Design review of the part built by this model. Coordinates are the model's own, in mm. A direction names the side the tool comes from. Coordinates: 2 decimals unless noted, no trailing zeros. Loops run counter-clockwise (first coordinate to the right, second up) from the corner with the lowest first, then second, coordinate; pieces in that order, holes last. Notation, with made-up numbers: (29.25, -3) -> (60.25, -3) arc R34 ccw to (60.25, 30) -> close; hole circle Ø2 at (-1, 67). An arc over 180 degrees is marked (long way). One line per item, written item: value. Start each with the question number.
1. Add section C-C on y = 22. Write out the cut boundary in (x, z), plus the area to 3 significant figures.
2. Draft analysis for pull direction X (two halves, no side actions). For faces 3 (the flat face through (2, 19, 7.62)), 4 (the flat face through (-93.294, 17, 15)), 5 (the cylindrical face through (98.219, -52.015, 15.382)), 6 (the flat face through (94.666, 85, 15)), state which applies: pulls with the +X half, pulls with the -X half, needs draft (parallel to the pull), parting line crosses it, or undercut.
3. Add section B-B on x = 80.5. Write out the cut boundary in (y, z), plus the area to 3 significant figures.
4. Machinability: for faces 1 (the cylindrical face through (4.506, -52.015, 1.528)), 2 (the flat face through (4, 81.156, 6)), which of the approach directions +Z, -Z, +X, -X, +Y, -Y give a long, thin tool a straight path to every point of the face, cutting with its end or side? Answer none if there is none.
5. Add section A-A on z = 17.75. Write out the cut boundary in (x, y), plus the area to 3 significant figures.
6. Insertion check: pin 1 (1.5 mm diameter, centred on x = 50, z = 13, fed in from +Y); pin 2 (12 mm diameter, centred on x = 79, y = -39, fed in from +Z). Each pin has a flat end and moves straight along its axis. Give the tip position at first contact, or say it passes through.
7. For probe 1 along X at (y, z) = (41, 15); probe 2 along Z at (x, y) = (22, 2); probe 3 along Y at (x, z) = (36, 7.75), list the stretches that pass through material, from the lowest coordinate up.
```python
from build123d import *

# Parameters (mm, degrees)
F0_W      = 193.04
F0_H      = 142.24
F1_DEPTH  = 25.4
F2_T      = -7.62
F3_R      = 5.08
F1_FACE_W = 182.88
F1_FACE_H = 20.32
F4_DEPTH  = 7.62


with BuildPart() as f1:
    # F0 (on Top) → F1 (new body)
    with BuildSketch(Plane.XY):
        with Locations((3.226209, 17.656468)):
            Rectangle(F0_W, F0_H)
    extrude(amount=F1_DEPTH)

    # F2
    f2_openings = [f1.faces().sort_by_distance(p)[0] for p in [
        (3.226209, 17.656468, 25.4),
    ]]
    offset(amount=F2_T, openings=f2_openings)

    # F3
    f3_edges = [f1.edges().sort_by_distance(p)[0] for p in [
        (-93.293791, -53.463532, 12.7),
        (-93.293791, 88.776468, 12.7),
        (99.746209, 88.776468, 12.7),
        (99.746209, -53.463532, 12.7),
        (3.226209, 88.776468, 0),
        (99.746209, 17.656468, 0),
        (3.226209, -53.463532, 0),
        (-93.293791, 17.656468, 0),
    ]]
    fillet(f3_edges, radius=F3_R)

    # F1_face (on face) → F4 (cut)
    with BuildSketch(Plane(origin=(3.226209, 88.776468, 15.24), x_dir=(-1, 0, 0), z_dir=(0, 1, 0))):
        Rectangle(F1_FACE_W, F1_FACE_H)
    extrude(amount=-F4_DEPTH, mode=Mode.SUBTRACT)


solid = f1.part
```
Worked answers:
1. outline: (-93.29, 5.08) arc R5.08 ccw to (-88.21, 0) -> (94.67, 0) arc R5.08 ccw to (99.75, 5.08) -> (99.75, 25.4) -> (92.13, 25.4) -> (92.13, 7.62) -> (-85.67, 7.62) -> (-85.67, 25.4) -> (-93.29, 25.4) -> close
1. area: 1,730 mm²
2. face 3: undercut
2. face 4: pulls with the -X half
2. face 5: pulls with the +X half
2. face 6: undercut
3. outline: (-53.46, 5.08) arc R5.08 ccw to (-48.38, 0) -> (83.7, 0) arc R5.08 ccw to (88.78, 5.08) -> (81.16, 5.08) -> (81.16, 7.62) -> (-45.84, 7.62) -> (-45.84, 25.4) -> (-53.46, 25.4) -> close
3. area: 1,190 mm²
4. face 1: -Z, +X, -X, -Y
4. face 2: +Z, +Y
5. outline: (-93.29, -48.38) arc R5.08 ccw to (-88.21, -53.46) -> (94.67, -53.46) arc R5.08 ccw to (99.75, -48.38) -> (99.75, 83.7) arc R5.08 ccw to (94.67, 88.78) -> (94.67, 81.16) -> (92.13, 81.16) -> (92.13, -45.84) -> (-85.67, -45.84) -> (-85.67, 81.16) -> (-88.21, 81.16) -> (-88.21, 88.78) arc R5.08 ccw to (-93.29, 83.7) -> close
5. area: 3,460 mm²
6. pin 1: stops at y = -45.84
6. pin 2: stops at z = 7.62
7. probe 1: x = -93.29 to -85.67, 92.13 to 99.75
7. probe 2: z = 0 to 7.62
7. probe 3: y = -53.46 to -45.84
